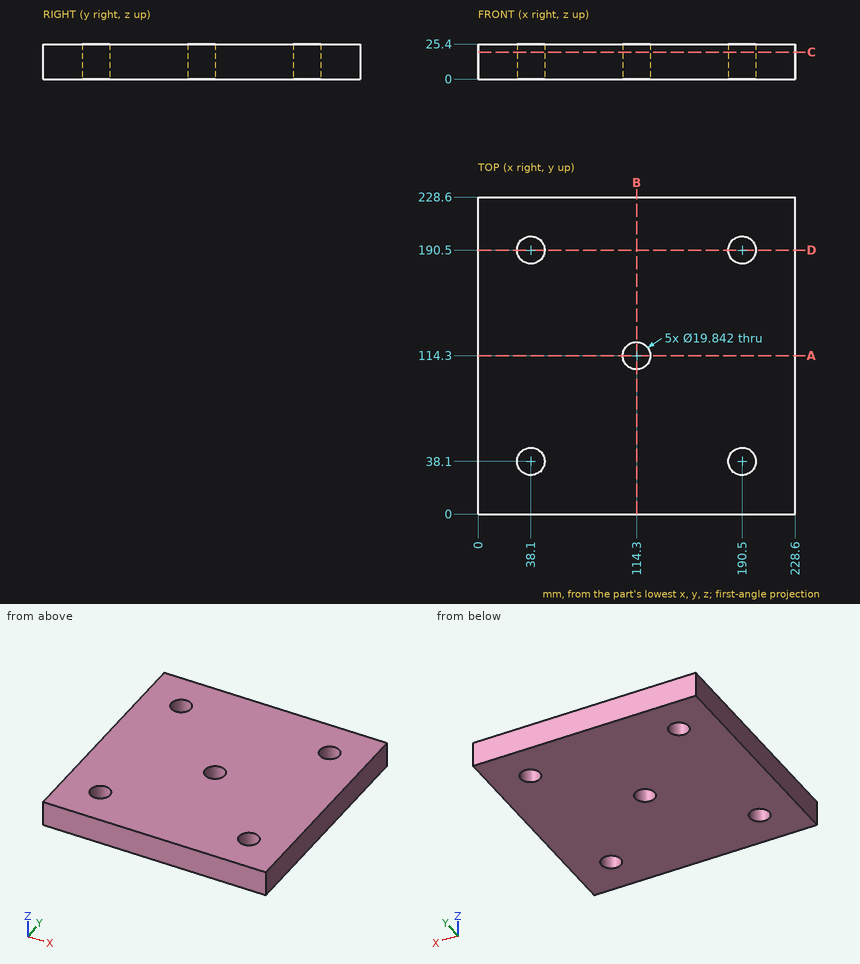
Print and shaded views of the part. All mm, measured from the part's lowest x, y and z. Give positions to 0.01 mm unless a question says otherwise; leave off trailing zeros. Loops run counter-clockwise (first coordinate to the right, second up) from the corner with the lowest first, then second, coordinate; pieces in that order, holes last.
1) Saw through at C-C (z = 19.5). Write the cut outline in (x, y).
2) Wall check: line 1 (Y direction, x = 38.1, z = 9.5); line 2 (Y direction, x = 114.3, z = 9); line 3 (Y direction, x = 192, z = 24.75). Give the ranges that are in metal, low to high.
3) Saw through at A-A (y = 114.3). Write the cut outline in (x, z), plus the area to 3 significant figures.
4) Saw through at D-D (y = 190.5). Write the cut outline in (x, z), plus the area to 3 significant figures.
5) Flat gauge pin, fed straight in: pin 1 Ø23 at (x, y) = (190.5, 190.5) entering from -Z. Where does the tip first touch, or does it go through?
Answer block:
1. outline: (0, 0) - (228.6, 0) - (228.6, 228.6) - (0, 228.6) - close; hole circle Ø19.84 at (38.1, 38.1); hole circle Ø19.84 at (38.1, 190.5); hole circle Ø19.84 at (114.3, 114.3); hole circle Ø19.84 at (190.5, 38.1); hole circle Ø19.84 at (190.5, 190.5)
2. line 1: y = 0 to 28.18, 48.02 to 180.58, 200.42 to 228.6
2. line 2: y = 0 to 104.38, 124.22 to 228.6
2. line 3: y = 0 to 28.29, 47.91 to 180.69, 200.31 to 228.6
3. outline: (0, 0) - (104.38, 0) - (104.38, 25.4) - (0, 25.4) - close; (124.22, 0) - (228.6, 0) - (228.6, 25.4) - (124.22, 25.4) - close
3. area: 5,300 mm2
4. outline: (0, 0) - (28.18, 0) - (28.18, 25.4) - (0, 25.4) - close; (48.02, 0) - (180.58, 0) - (180.58, 25.4) - (48.02, 25.4) - close; (200.42, 0) - (228.6, 0) - (228.6, 25.4) - (200.42, 25.4) - close
4. area: 4,800 mm2
5. pin 1: stops at z = 0
